from build123d import *

# Parameters (mm, degrees)
F1_DEPTH = 3


with BuildPart() as f1:
    # F0 (on Top) → F1 (new body)
    with BuildSketch(Plane.XY):
        with BuildLine():
            Line((3.5, 50), (-3.5, 50))
            ThreePointArc((-3.5, 50), (-7.035534, 48.535534), (-8.5, 45))
            Line((-8.5, 45), (-8.5, 5))
            ThreePointArc((-8.5, 5), (-7.035534, 1.464466), (-3.5, 0))
            Line((-3.5, 0), (3.5, 0))
            ThreePointArc((3.5, 0), (7.035534, 1.464466), (8.5, 5))
            Line((8.5, 5), (8.5, 45))
            ThreePointArc((8.5, 45), (7.035534, 48.535534), (3.5, 50))
        make_face()
        with BuildLine():
            ThreePointArc((-6.5, 7.95), (-6.676777, 8.376777), (-6.25, 8.2))
            Line((-6.25, 8.2), (-3.25, 8.2))
            ThreePointArc((-3.25, 8.2), (-3, 8.45), (-2.75, 8.2))
            ThreePointArc((-2.75, 8.2), (-2.823223, 8.023223), (-3, 7.95))
            Line((-3, 7.95), (-3, 5.25))
            ThreePointArc((-3, 5.25), (-2.823223, 5.176777), (-2.75, 5))
            ThreePointArc((-2.75, 5), (-3, 4.75), (-3.25, 5))
            Line((-3.25, 5), (-6.25, 5))
            ThreePointArc((-6.25, 5), (-6.676777, 4.823223), (-6.5, 5.25))
            Line((-6.5, 5.25), (-6.5, 7.95))
        make_face(mode=Mode.SUBTRACT)
        with BuildLine():
            ThreePointArc((-2.75, 18.2), (-2.823223, 18.023223), (-3, 17.95))
            Line((-3, 17.95), (-3, 15.25))
            ThreePointArc((-3, 15.25), (-2.823223, 15.176777), (-2.75, 15))
            ThreePointArc((-2.75, 15), (-3, 14.75), (-3.25, 15))
            Line((-3.25, 15), (-6.25, 15))
            ThreePointArc((-6.25, 15), (-6.676777, 14.823223), (-6.5, 15.25))
            Line((-6.5, 15.25), (-6.5, 17.95))
            ThreePointArc((-6.5, 17.95), (-6.676777, 18.376777), (-6.25, 18.2))
            Line((-6.25, 18.2), (-3.25, 18.2))
            ThreePointArc((-3.25, 18.2), (-3, 18.45), (-2.75, 18.2))
        make_face(mode=Mode.SUBTRACT)
        with BuildLine():
            ThreePointArc((-1, 7.95), (-1.176777, 8.376777), (-0.75, 8.2))
            Line((-0.75, 8.2), (0.75, 8.2))
            ThreePointArc((0.75, 8.2), (1, 8.45), (1.25, 8.2))
            ThreePointArc((1.25, 8.2), (1.176777, 8.023223), (1, 7.95))
            Line((1, 7.95), (1, 5.25))
            ThreePointArc((1, 5.25), (1.176777, 5.176777), (1.25, 5))
            ThreePointArc((1.25, 5), (1, 4.75), (0.75, 5))
            Line((0.75, 5), (-0.75, 5))
            ThreePointArc((-0.75, 5), (-1.176777, 4.823223), (-1, 5.25))
            Line((-1, 5.25), (-1, 7.95))
        make_face(mode=Mode.SUBTRACT)
        with BuildLine():
            ThreePointArc((3, 7.95), (2.823223, 8.376777), (3.25, 8.2))
            Line((3.25, 8.2), (6.25, 8.2))
            ThreePointArc((6.25, 8.2), (6.5, 8.45), (6.75, 8.2))
            ThreePointArc((6.75, 8.2), (6.676777, 8.023223), (6.5, 7.95))
            Line((6.5, 7.95), (6.5, 5.25))
            ThreePointArc((6.5, 5.25), (6.676777, 5.176777), (6.75, 5))
            ThreePointArc((6.75, 5), (6.5, 4.75), (6.25, 5))
            Line((6.25, 5), (3.25, 5))
            ThreePointArc((3.25, 5), (2.823223, 4.823223), (3, 5.25))
            Line((3, 5.25), (3, 7.95))
        make_face(mode=Mode.SUBTRACT)
        with BuildLine():
            ThreePointArc((1.25, 18.2), (1.176777, 18.023223), (1, 17.95))
            Line((1, 17.95), (1, 15.25))
            ThreePointArc((1, 15.25), (1.176777, 15.176777), (1.25, 15))
            ThreePointArc((1.25, 15), (1, 14.75), (0.75, 15))
            Line((0.75, 15), (-0.75, 15))
            ThreePointArc((-0.75, 15), (-1.176777, 14.823223), (-1, 15.25))
            Line((-1, 15.25), (-1, 17.95))
            ThreePointArc((-1, 17.95), (-1.176777, 18.376777), (-0.75, 18.2))
            Line((-0.75, 18.2), (0.75, 18.2))
            ThreePointArc((0.75, 18.2), (1, 18.45), (1.25, 18.2))
        make_face(mode=Mode.SUBTRACT)
        with BuildLine():
            ThreePointArc((3, 17.95), (2.823223, 18.376777), (3.25, 18.2))
            Line((3.25, 18.2), (6.25, 18.2))
            ThreePointArc((6.25, 18.2), (6.5, 18.45), (6.75, 18.2))
            ThreePointArc((6.75, 18.2), (6.676777, 18.023223), (6.5, 17.95))
            Line((6.5, 17.95), (6.5, 15.25))
            ThreePointArc((6.5, 15.25), (6.676777, 15.176777), (6.75, 15))
            ThreePointArc((6.75, 15), (6.5, 14.75), (6.25, 15))
            Line((6.25, 15), (3.25, 15))
            ThreePointArc((3.25, 15), (2.823223, 14.823223), (3, 15.25))
            Line((3, 15.25), (3, 17.95))
        make_face(mode=Mode.SUBTRACT)
        with BuildLine():
            ThreePointArc((-3.25, 45), (-3, 45.25), (-2.75, 45))
            ThreePointArc((-2.75, 45), (-2.823223, 44.823223), (-3, 44.75))
            Line((-3, 44.75), (-3, 42.05))
            ThreePointArc((-3, 42.05), (-2.823223, 41.976777), (-2.75, 41.8))
            ThreePointArc((-2.75, 41.8), (-3, 41.55), (-3.25, 41.8))
            Line((-3.25, 41.8), (-6.25, 41.8))
            ThreePointArc((-6.25, 41.8), (-6.676777, 41.623223), (-6.5, 42.05))
            Line((-6.5, 42.05), (-6.5, 44.75))
            ThreePointArc((-6.5, 44.75), (-6.676777, 45.176777), (-6.25, 45))
            Line((-6.25, 45), (-3.25, 45))
        make_face(mode=Mode.SUBTRACT)
        with BuildLine():
            ThreePointArc((-1, 44.75), (-1.176777, 45.176777), (-0.75, 45))
            Line((-0.75, 45), (0.75, 45))
            ThreePointArc((0.75, 45), (1, 45.25), (1.25, 45))
            ThreePointArc((1.25, 45), (1.176777, 44.823223), (1, 44.75))
            Line((1, 44.75), (1, 42.05))
            ThreePointArc((1, 42.05), (1.176777, 41.976777), (1.25, 41.8))
            ThreePointArc((1.25, 41.8), (1, 41.55), (0.75, 41.8))
            Line((0.75, 41.8), (-0.75, 41.8))
            ThreePointArc((-0.75, 41.8), (-1.176777, 41.623223), (-1, 42.05))
            Line((-1, 42.05), (-1, 44.75))
        make_face(mode=Mode.SUBTRACT)
        with BuildLine():
            ThreePointArc((6.25, 45), (6.5, 45.25), (6.75, 45))
            ThreePointArc((6.75, 45), (6.676777, 44.823223), (6.5, 44.75))
            Line((6.5, 44.75), (6.5, 42.05))
            ThreePointArc((6.5, 42.05), (6.676777, 41.976777), (6.75, 41.8))
            ThreePointArc((6.75, 41.8), (6.5, 41.55), (6.25, 41.8))
            Line((6.25, 41.8), (3.25, 41.8))
            ThreePointArc((3.25, 41.8), (2.823223, 41.623223), (3, 42.05))
            Line((3, 42.05), (3, 44.75))
            ThreePointArc((3, 44.75), (2.823223, 45.176777), (3.25, 45))
            Line((3.25, 45), (6.25, 45))
        make_face(mode=Mode.SUBTRACT)
    extrude(amount=F1_DEPTH)


solid = f1.part
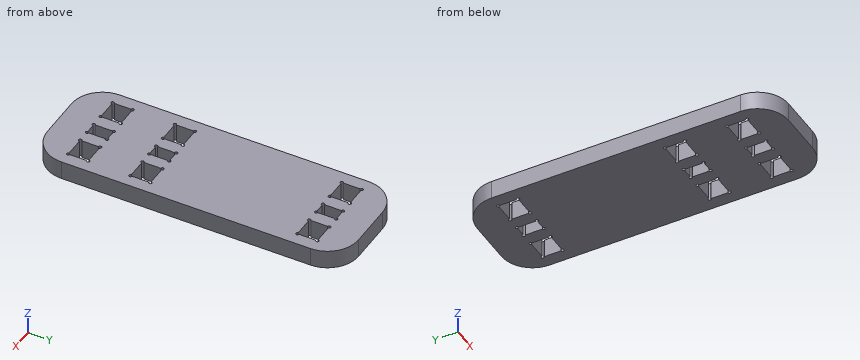
Geometry check sheet. Reference: the model listing, model coordinates, mm. Give positions to 0.01 mm unless a question says otherwise; leave off trailing zeros. Loops run counter-clockwise (first coordinate to the right, second up) from the corner with the lowest first, then second, coordinate; pieces in that order, holes last. Notation, with made-up numbers: M 18,80.5 L 56,80.5 A30 cw 56,102.5 Z; hole C 5.5,66 d6. An arc over 180 degrees is marked long. Answer as a JSON object with one key per item and string values. Group by question number.
Item 1: Sectioned sample at B-B on z = 1.5. Give the number of separate pieces and of enclosed holes in the cut face, plus the area to 3 significant figures.
Item 2: Gauge pin test, flat end, axial feed: pin 1 (1 mm diameter, centred on x = 5, z = 1, fed in from -Y). Record the tip position at first contact, or that the pin passes through.
Item 3: Sectioned sample at A-A on x = -5.5. Record the boundary of the cut face in (y, z), plus the area to 3 significant figures.
Item 4: Material ranges on L1, parallel to Y at x = 0.25, z = 1.9; L2, parallel to Y at x = -5, z = 2; L3, parallel to X at y = 3.5, z = 2.9, recorded low to high.
Findings below:
{
 "1": {"separate pieces": "1", "enclosed holes": "9", "area": "737 mm2"},
 "2": {"pin 1": "y = 0.1"},
 "3": {"outline": "M 0.42,0 L 5,0 L 5,3 L 0.42,3 Z; M 8.2,0 L 15,0 L 15,3 L 8.2,3 Z; M 18.2,0 L 41.8,0 L 41.8,3 L 18.2,3 Z; M 45,0 L 49.58,0 L 49.58,3 L 45,3 Z", "area": "119 mm2"},
 "4": {"L1": "0 to 5, 8.2 to 15, 18.2 to 41.8, 45 to 50", "L2": "0.23 to 5, 8.2 to 15, 18.2 to 41.8, 45 to 49.77", "L3": "-8.27 to 8.27"}
}
